Check sheet for the modelled part. Datum: model origin and axes. Units: mm. Face numbers are marked on the shaded views. A direction names the side the tool comes from. Round coordinates to 2 decimals unless told otherwise and drop trailing zeros. Write each loop counter-clockwise with the first axis right and the second up, starting at its lowest first coordinate (ties: lowest second). Pieces come first, ordered by that corner, then holes. Notation, with made-up numbers: M -39.5,-6 L -34.5,-6 A27 cw -34.5,17 Z; hole C 13,42 d9. An arc over 180 degrees is marked long. Answer in a Markdown table with one row per item.
```python
from build123d import *

# Parameters (mm, degrees)
F1_W     = 106
F1_H     = 8
F1_R     = 1.5
F2_DEPTH = 27
F3_W     = 96
F3_H     = 23
F4_DEPTH = 25
F5_SIZE  = 3
F6_R     = 0.5


with BuildPart() as f2:
    # F1 (on Top) → F2 (new body)
    with BuildSketch(Plane.XY):
        Rectangle(F1_W, F1_H)
        with Locations((-37.5, 0)):
            Circle(F1_R, mode=Mode.SUBTRACT)
        with Locations((-27.5, 0)):
            Circle(F1_R, mode=Mode.SUBTRACT)
        Circle(F1_R, mode=Mode.SUBTRACT)
        with Locations((27.5, 0)):
            Circle(F1_R, mode=Mode.SUBTRACT)
        with Locations((37.5, 0)):
            Circle(F1_R, mode=Mode.SUBTRACT)
    extrude(amount=F2_DEPTH)

    # F3 (on face) → F4 (cut)
    with BuildSketch(Plane.XZ.offset(4)):
        with Locations((0, 13.5)):
            Rectangle(F3_W, F3_H)
    extrude(amount=-F4_DEPTH, mode=Mode.SUBTRACT)

    # F5
    f5_edges = [f2.edges().sort_by_distance(p)[0] for p in [
        (-53, 0, 27),
        (53, 0, 27),
    ]]
    chamfer(f5_edges, length=F5_SIZE)

    # F6
    f6_edges = [f2.edges().sort_by_distance(p)[0] for p in [
        (0, -4, 27),
        (0, 4, 27),
        (51.5, -4, 25.5),
        (53, -4, 12),
        (51.5, 4, 25.5),
        (53, 4, 12),
        (-51.5, -4, 25.5),
        (-51.5, 4, 25.5),
        (-53, -4, 12),
        (-53, 4, 12),
    ]]
    fillet(f6_edges, radius=F6_R)


solid = f2.part
```
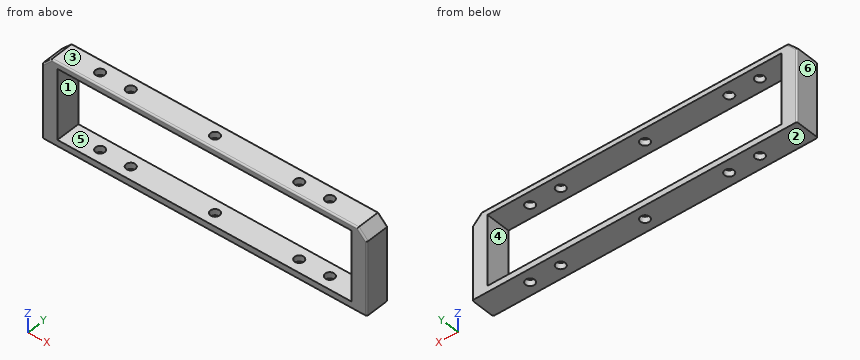
1. Section check C-C, the plane z = 5.5. Record the cut outline in (x, y).
Found:
| item | result |
|---|---|
| outline | M -53,-3.5 A0.5 ccw -52.5,-4 L -48,-4 L -48,4 L -52.5,4 A0.5 ccw -53,3.5 Z; M 48,-4 L 52.5,-4 A0.5 ccw 53,-3.5 L 53,3.5 A0.5 ccw 52.5,4 L 48,4 Z |
2. Access from +Z, -Z, +X, -X, +Y, -Y to the whole of each face (thin tool, end or side, straight path). Record for the marked faces 1 and 2.
Found:
| item | result |
|---|---|
| face 1 | +Y, -Y |
| face 2 | -Z, +X, -X, +Y, -Y |
3. Draft check along Z on the marked faces 3, 4, 5 and 6. Enter one of: +Z half, -Z half, draft (parallel to the pull), parting line (faces both ways), or undercut.
Found:
| item | result |
|---|---|
| face 3 | +Z half |
| face 4 | undercut |
| face 5 | undercut |
| face 6 | draft |
4. Section check B-B, the plane y = -2.5. Record the cut outline in (x, z), and give its area (3 significant figures).
Found:
| item | result |
|---|---|
| outline | M -53,0 L 53,0 L 53,24 L 50,27 L -50,27 L -53,24 Z; hole M -48,2 L 48,2 L 48,25 L -48,25 Z |
| area | 645 mm2 |
5. Scan lines: L1, parallel to X at y = 0, z = 1.55; L2, parallel to Z at x = 35, y = 3.5; L3, parallel to X at y = 0, z = 25.85. Record each from-to range of solid material in increasing order.
Found:
| item | result |
|---|---|
| L1 | x = -53 to -39, -36 to -29, -26 to -1.5, 1.5 to 26, 29 to 36, 39 to 53 |
| L2 | z = 0 to 2, 25 to 27 |
| L3 | x = -51.15 to -39, -36 to -29, -26 to -1.5, 1.5 to 26, 29 to 36, 39 to 51.15 |
6. Section check D-D, the plane x = 27.5. Record the cut outline in (y, z).
Found:
| item | result |
|---|---|
| outline | M -4,0 L -1.5,0 L -1.5,2 L -4,2 Z; M -4,25 L -1.5,25 L -1.5,27 L -3.5,27 A0.5 ccw -4,26.5 Z; M 1.5,0 L 4,0 L 4,2 L 1.5,2 Z; M 1.5,25 L 4,25 L 4,26.5 A0.5 ccw 3.5,27 L 1.5,27 Z |
7. Section check A-A, the plane x = -11.5. Record the cut outline in (y, z), and give its area (3 significant figures).
Found:
| item | result |
|---|---|
| outline | M -4,0 L 4,0 L 4,2 L -4,2 Z; M -4,25 L 4,25 L 4,26.5 A0.5 ccw 3.5,27 L -3.5,27 A0.5 ccw -4,26.5 Z |
| area | 31.9 mm2 |
